Source: three-view drawing plus pictorial views. Frame: mm from the lowest corner of the part. Coordinates: 2 decimals unless noted, no trailing zeros. Order: outer loops, then holes, each group sorted by start corner. A loop starts at its lowest first (then second) coordinate and runs counter-clockwise, first axis right, second up. Notation, with made-up numbers: (37.5, 16.25) - (51.5, 16.25) arc R33 cw to (51.5, 50.25) - close; hole circle Ø7 at (19, -15). An arc over 180 degrees is marked (long way). One line per question, with ' | ' between items.
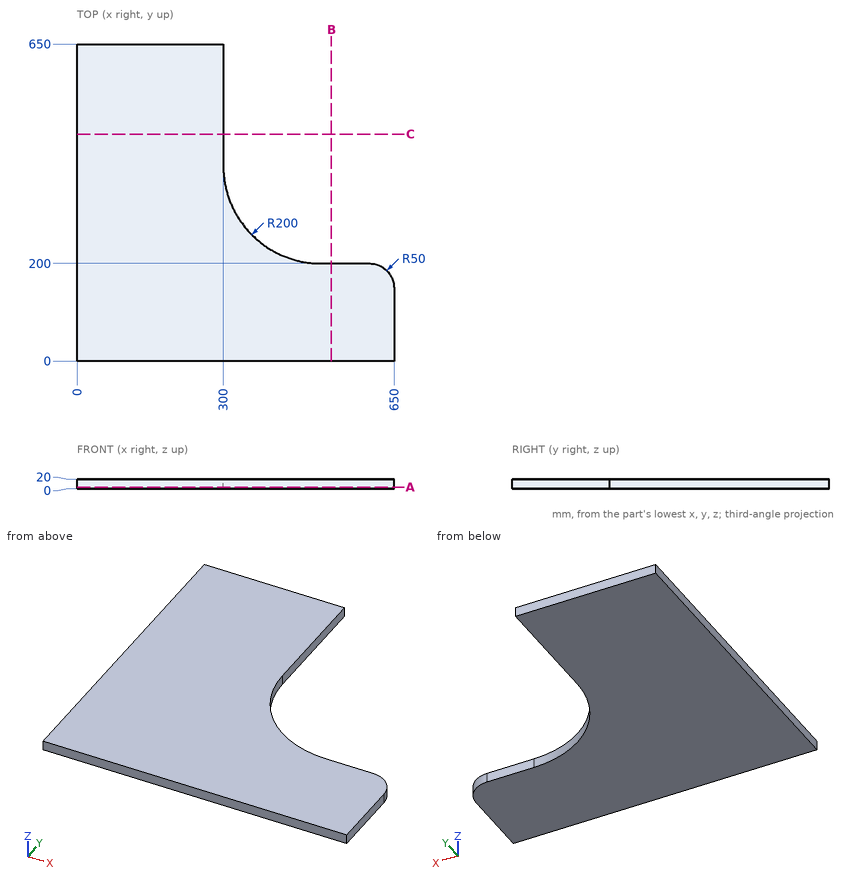
Item 1: Contact query for a flat-ended pin moving along its axis: P1, Ø6, axis at y = 478.5, z = 13, coming from the +X side. Output: stop coordinate, or through.
Data:
P1: x = 300
Item 2: Section B-B on x = 521.5. Return the cut outline in (y, z), and give its area (3 significant figures).
Data:
outline: (0, 0) - (200, 0) - (200, 20) - (0, 20) - close | area: 4,000 mm^2
Item 3: Section C-C on y = 465. Return the cut outline in (x, z), and give its area (3 significant figures).
Data:
outline: (0, 0) - (300, 0) - (300, 20) - (0, 20) - close | area: 6,000 mm^2
Item 4: Section A-A on z = 3.5. Return the cut outline in (x, y).
Data:
outline: (0, 0) - (650, 0) - (650, 150) arc R50 ccw to (600, 200) - (500, 200) arc R200 cw to (300, 400) - (300, 650) - (0, 650) - close
Item 5: Ray query, line 1 (X direction, y = 412.5, z = 4); line 2 (Y direction, x = 557, z = 2.25); line 3 (X direction, y = 356, z = 12.5). Return the intervals inside material, ascending.
Data:
line 1: 0 to 300 | line 2: 0 to 200 | line 3: 0 to 304.9
